Geometry: final body of the model. Coordinates: model frame, mm. A direction names the side the tool comes from. Round coordinates to 2 decimals unless told otherwise and drop trailing zeros. Loops run counter-clockwise (first coordinate to the right, second up) from the corner with the lowest first, then second, coordinate; pieces in that order, holes last. Notation, with made-up numbers: (28, 60) - (33, 60) arc R14 ccw to (33, 82) - close; hole circle Ø1 at (-14.5, -21.5). An arc over 180 degrees is marked (long way). Return JSON: item names as keys, results as strings. Group by question number.
1. First-contact query: pin 1 Ø1 at (x, z) = (-0.5, 0.5) entering from +Y; pin 2 Ø1 at (x, y) = (2.5, 3) entering from -Z. Flat tips, straight axial feed; report the tip coordinate or a pass-through.
2. Draft query along Z for faces 4 (the face through (2.003, 16.724, -0.631)), 5 (the face through (3.233, 14.604, 1.341)), 6 (the face through (-1, 0, 1)). Return one class per face: +Z half, -Z half, draft (parallel to the pull), parting line (faces both ways), or undercut.
3. Set-up query: faces 1 (the face through (0, 7.1, -2)), 2 (the face through (-3, 3, 0)), 3 (the face through (2, 21.9, -2)). Return all of +Z, -Z, +X, -X, +Y, -Y with unobstructed straight access to the full face (end or side cutting, diameter ignored); none if empty.
4. Section C-C on y = 16.5. Return loops of the section in (x, z).
5. Material intervals for probe 1 along Z at (x, y) = (0, 16.5); probe 2 along Y at (x, z) = (-1.25, 2); probe 3 along Z at (x, y) = (0, 3.25), sorted ascending.
6. Section B-B on z = 0. Return loops of the section in (x, y).
7. Section A-A on x = 0. Return loops of the section in (y, z), and give its area (3 significant figures).
8. Section D-D on z = -2.5. Return loops of the section in (x, y), and give its area (3 significant figures).
Autodesk Inventor part; units mm, degrees
ref_plane "YZ Plane" through (0, 0, 0) normal (1, 0, 0) x (0, 1, 0)
ref_plane "XZ Plane" through (0, 0, 0) normal (0, 1, 0) x (-1, 0, 0)
ref_plane "XY Plane" through (0, 0, 0) normal (0, 0, 1) x (1, 0, 0)
sketch "Sketch1" plane through (0, 0, 0) normal (0, 0, 1) x (1, 0, 0)
  line L0 (0, 0) -> (3, 0)
  line L1 (3, 0) -> (3, 5)
  line L2 (3, 5) -> (1.4, 5)
  line L3 (1.4, 5) -> (1.4, 7.1)
  line L4 (1.4, 7.1) -> (3.5, 7.1)
  line L5 (3.5, 7.1) -> (3.5, 21.9)
  line L6 (3.5, 21.9) -> (0, 21.9)
  line L7 (0, 21.9) -> (0, 0)
  dimension "d0" = 3
  dimension "d1" = 5
  dimension "d2" = 1.4
  dimension "d3" = 2.1
  dimension "d4" = 3.5
  dimension "d5" = 14.8
revolve "Revolution1" add sketch "Sketch1" angle 360 about axis through (0, 21.9, 0) along (0, -1, 0)
thread "Thread1"
thread "Thread2"
sketch "Sketch2" plane through (0, 0, 0) normal (0, -1, 0) x (1, 0, 0)
  circle A0 centre (0, 0) radius 3.5
  circle A1 centre (0, 0) radius 1
  dimension "d11" = 2
extrude "Extrusion1" cut sketch "Sketch2" against normal up to surface (21.9 mm away) contours A1
sketch "Sketch3" plane through (0, 21.9, 0) normal (0, 1, 0) x (1, 0, 0)
  circle A0 centre (0, 0) radius 1
  circle A1 centre (0, 0) radius 3.5
  circle A2 centre (0, 0) radius 2.1
  dimension "d14" = 4.2
extrude "Extrusion2" cut sketch "Sketch3" against normal blind 10.5 contours A2
properties part number "E3DV6HeatBreak" material "Stainless Steel"
Taken from the geometry:
{
 "1": {"pin 1": "y = 11.4", "pin 2": "z = -2.24"},
 "2": {"face 4": "undercut", "face 5": "parting line", "face 6": "draft"},
 "3": {"face 1": "none", "face 2": "-Y", "face 3": "+Z, -Z, +X, -X, +Y"},
 "4": {"outline": "circle Ø7 at (0, 0); hole circle Ø4.2 at (0, 0)"},
 "5": {"probe 1": "-3.5 to -2.1, 2.1 to 3.5", "probe 2": "0 to 5, 7.1 to 21.9", "probe 3": "-3 to -1, 1 to 3"},
 "6": {"outline": "(-3.5, 7.1) - (-1.4, 7.1) - (-1.4, 5) - (-3, 5) - (-3, 0) - (-1, 0) - (-1, 11.4) - (-2.1, 11.4) - (-2.1, 21.9) - (-3.5, 21.9) - close; (1, 0) - (3, 0) - (3, 5) - (1.4, 5) - (1.4, 7.1) - (3.5, 7.1) - (3.5, 21.9) - (2.1, 21.9) - (2.1, 11.4) - (1, 11.4) - close"},
 "7": {"outline": "(0, -3) - (5, -3) - (5, -1.4) - (7.1, -1.4) - (7.1, -3.5) - (21.9, -3.5) - (21.9, -2.1) - (11.4, -2.1) - (11.4, -1) - (0, -1) - close; (0, 1) - (11.4, 1) - (11.4, 2.1) - (21.9, 2.1) - (21.9, 3.5) - (7.1, 3.5) - (7.1, 1.4) - (5, 1.4) - (5, 3) - (0, 3) - close", "area": "72.6 mm2"},
 "8": {"outline": "(-2.45, 7.1) - (2.45, 7.1) - (2.45, 21.9) - (-2.45, 21.9) - close; (-1.66, 0) - (1.66, 0) - (1.66, 5) - (-1.66, 5) - close", "area": "89.1 mm2"}
}
